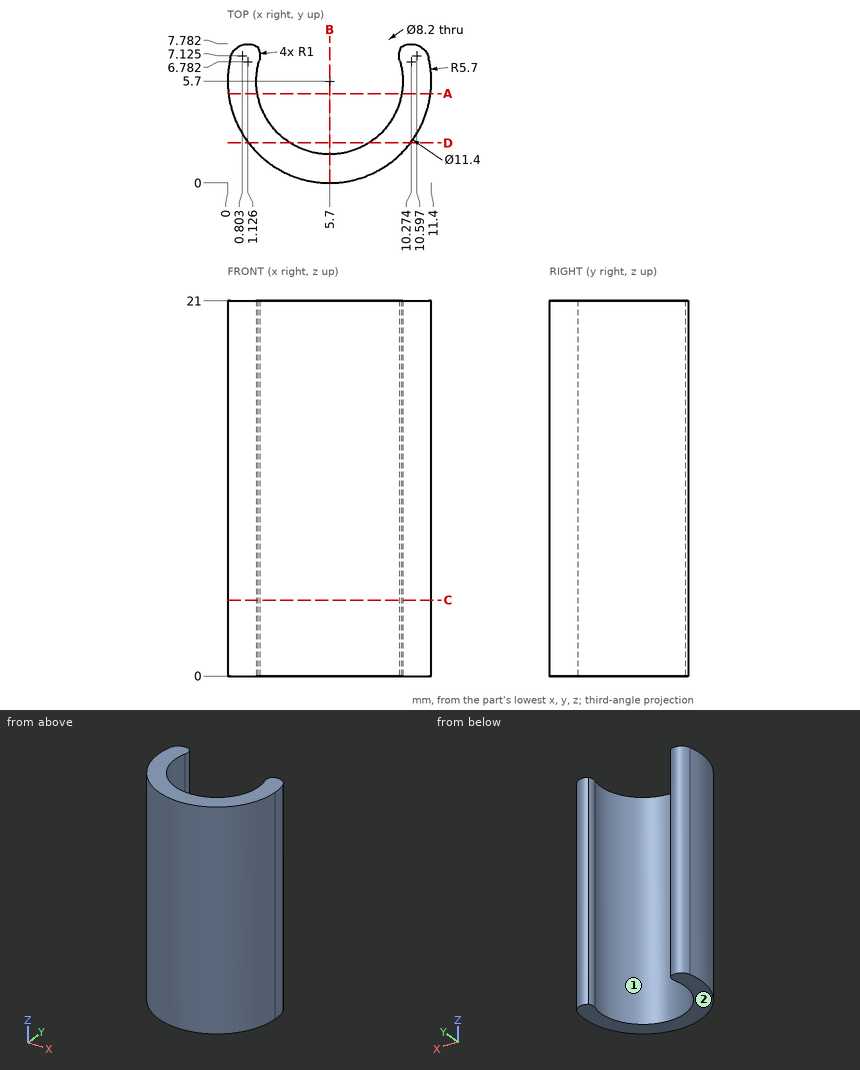
Geometry: see drawing. Coordinates: mm, zero at the bounding-box minimum. Give positions to 0.01 mm unless a question says otherwise; leave off trailing zeros. Order: outer loops, then holes, each group sorted by start corner. A loop starts at its lowest first (then second) coordinate and runs counter-clockwise, first axis right, second up. Notation, with made-up numbers: (1, -34) - (7, -34) arc R24 cw to (7, -6) - close; hole circle Ø2 at (30.5, 78.25). An arc over 180 degrees is marked (long way). Use CSV: the item, a comma, the result in double quotes.
1. Section query D-D (y = 2.25). Output: boundary loops of the cut face in (x, z) (1 decimal).
Answers below:
outline,"(1.2, 0) - (3.5, 0) - (3.5, 21) - (1.2, 21) - close; (7.9, 0) - (10.2, 0) - (10.2, 21) - (7.9, 21) - close"
2. Material intervals for line 1 along X through (y, z) = (5.7, 12); line 2 along Y through (x, z) = (5.7, 15.75); line 3 along X through (y, z) = (3.5, 2.5), sorted ascending. Write a range as from..to.
Answers below:
line 1,"0..1.6, 9.8..11.4"
line 2,"0..1.6"
line 3,"0.44..2.24, 9.16..10.96"
3. Contact query for flat-ended pins moving along their axis: pin 1 (1 mm diameter, centred on y = 4, z = 16.5, fed in from -X); pin 2 (1.5 mm diameter, centred on x = 7, z = 12, fed in from +Y); pin 3 (2 mm diameter, centred on x = 3, z = 9, fed in from -Y). Output: stop coordinate, or through.
Answers below:
pin 1,"x = 0.13"
pin 2,"y = 2.15"
pin 3,"y = 0.26"
4. Section query B-B (x = 5.7). Output: boundary loops of the cut face in (y, z), plus the area to 3 significant figures.
Answers below:
outline,"(0, 0) - (1.6, 0) - (1.6, 21) - (0, 21) - close"
area,"33.6 mm2"
5. Section query C-C (z = 4.25). Output: boundary loops of the cut face in (x, y) (1 decimal).
Answers below:
outline,"(0.2, 7) arc R5.7 ccw (long way) to (11.2, 7) arc R1 ccw to (9.7, 7.6) arc R1 ccw to (9.6, 6.8) arc R4.1 cw (long way) to (1.8, 6.8) arc R1 ccw to (1.7, 7.6) arc R1 ccw to start"
6. Mould query, pull axis X, two halves, no side actions, for the marked faces 1 and 2. Classes: +X half, -X half, draft (parallel to the pull), parting line (faces both ways), or undercut.
Answers below:
face 1,"undercut"
face 2,"draft"
7. Section query A-A (y = 5). Output: boundary loops of the cut face in (x, z).
Answers below:
outline,"(0.04, 0) - (1.66, 0) - (1.66, 21) - (0.04, 21) - close; (9.74, 0) - (11.36, 0) - (11.36, 21) - (9.74, 21) - close"
